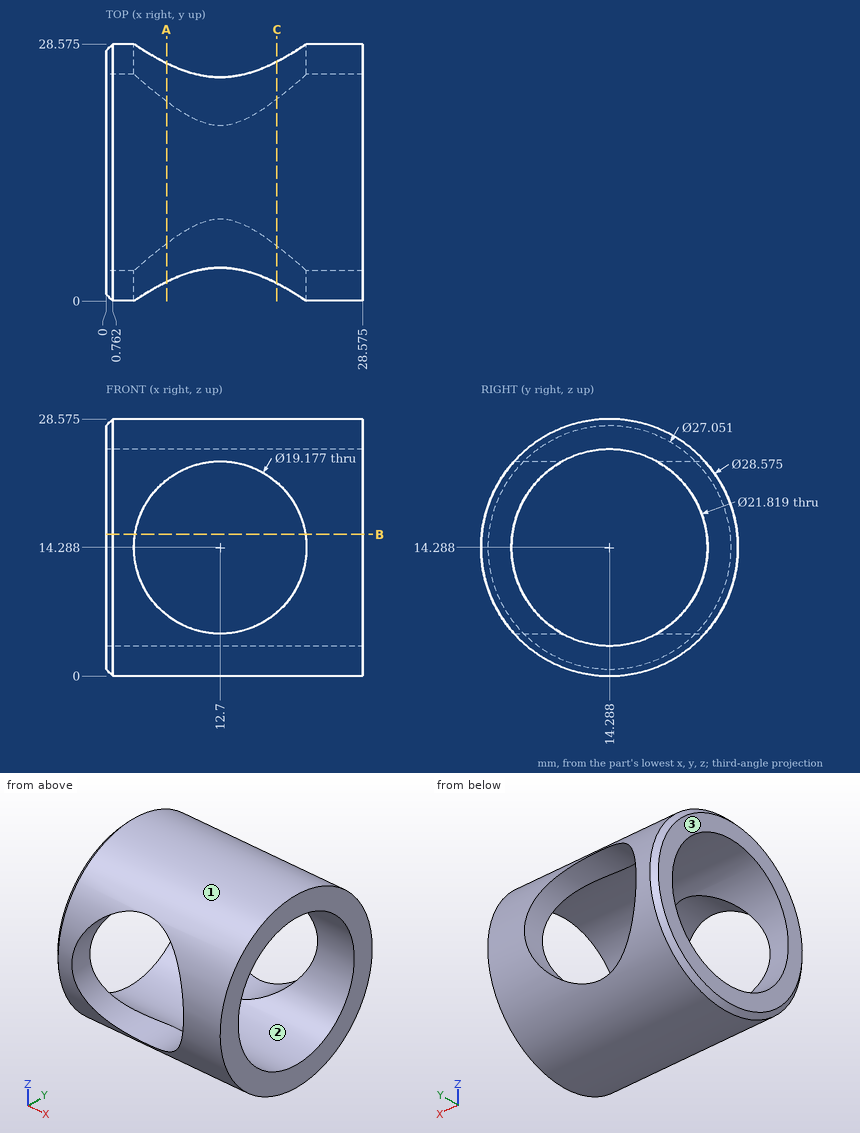
For this review, use the dimensioned drawing (mm, ordinates from the lowest corner) and the shaded views. Coordinates: 2 decimals unless noted, no trailing zeros. Write each loop counter-clockwise with the first axis right and the second up, starting at its lowest first coordinate (ties: lowest second). Pieces come first, ordered by that corner, then holes. Notation, with made-up numbers: (34.5, 2) -> (72.5, 2) arc R20 cw to (72.5, 31) -> close; hole circle Ø5 at (46.5, -34.75). An arc over 180 degrees is marked (long way). Put each result on its own line as item: value.
Q1. Wall thickness on L1, parallel to Y at x = 23.25, z = 14.75; L2, parallel to X at y = 25.25, z = 20.75 (1 decimal); L3, parallel to Z at x = 16.25, y = 17.25 (1 decimal): over which ranges is each line inside the solid? List them lowest first.
From the geometry:
L1: y = 0.01 to 3.39, 25.19 to 28.57
L2: x = 0 to 5.6, 19.8 to 28.6
L3: z = 0.3 to 3.8, 24.8 to 28.3
Q2. Take a section at A-A, the plane x = 6.75. State the section outline as (y, z) points (1 decimal), then the cut area to 3 significant figures.
From the geometry:
outline: (2.1, 6.8) arc R14.3 ccw to (26.4, 6.8) -> (22.2, 6.8) arc R10.9 cw to (6.4, 6.8) -> close; (2.1, 21.8) -> (6.4, 21.8) arc R10.9 cw to (22.2, 21.8) -> (26.4, 21.8) arc R14.3 ccw to start
area: 158 mm2
Q3. The part is to be moulded in two halves that separate along Y. For the marked faces 1, 2 and 3, say which applies: +Y half, -Y half, draft (parallel to the pull), parting line (faces both ways), or undercut.
From the geometry:
face 1: parting line
face 2: undercut
face 3: draft
Q4. Take a section at C-C, the plane x = 19. State the section outline as (y, z) points (1 decimal), then the cut area to 3 significant figures.
From the geometry:
outline: (2, 7.1) arc R14.3 ccw to (26.6, 7.1) -> (22.5, 7.1) arc R10.9 cw to (6.1, 7.1) -> close; (2, 21.5) -> (6.1, 21.5) arc R10.9 cw to (22.5, 21.5) -> (26.6, 21.5) arc R14.3 ccw to start
area: 163 mm2
Q5. Take a section at B-B, the plane z = 15.75. Count the separate pieces of the cut face and the enclosed holes in it.
From the geometry:
separate pieces: 4
enclosed holes: 0
Q6. Clearance check with flat-ended pins moving along their axes: pin 1 Ø5 at (y, z) = (15.5, 8) entering from +X; pin 2 Ø10 at (x, y) = (20, 19.5) entering from +Z; pin 3 Ø5 at (x, z) = (7, 7) entering from +Y; pin 4 Ø10 at (x, y) = (20, 23.5) entering from +Z. State where each tip first meets the part, or that it passes through.
From the geometry:
pin 1: passes through
pin 2: stops at z = 28.57
pin 3: stops at y = 27.37
pin 4: stops at z = 27.94
